from build123d import *

# Parameters (mm, degrees)
EXTRUDE_1_DEPTH        = 4
HOLE_WIZARD_M8_1_D     = 6.8
HOLE_WIZARD_M8_1_DEPTH = 19.75
HOLE_WIZARD_M8_1_TIP   = 2.042926105
FILLET_1_R             = 0.5


with BuildPart() as part:
    # 草图1 → 凸台-拉伸1 (new body)
    with BuildSketch(Plane.XY):
        Polygon((10.5, 14), (0, 0), (13.125, 0), (23.625, 14), align=None)
    extrude(amount=EXTRUDE_1_DEPTH)

    # M8 螺纹孔1
    with Locations(Plane(origin=(11.8125, 7, 4), x_dir=(1, 0, 0), z_dir=(0, 0, 1))):
        with Locations((0, 0)):
            Hole(HOLE_WIZARD_M8_1_D / 2, depth=HOLE_WIZARD_M8_1_DEPTH)
            with Locations((0, 0, -(HOLE_WIZARD_M8_1_DEPTH + HOLE_WIZARD_M8_1_TIP / 2))):  # 118° drill point
                Cone(0, HOLE_WIZARD_M8_1_D / 2, HOLE_WIZARD_M8_1_TIP, mode=Mode.SUBTRACT)

    # 圆角1
    fillet_1_edges = [part.edges().sort_by_distance(p)[0] for p in [
        (6.5625, 0, 4),
        (17.0625, 14, 4),
        (6.5625, 0, 0),
        (17.0625, 14, 0),
    ]]
    fillet(fillet_1_edges, radius=FILLET_1_R)


solid = part.part
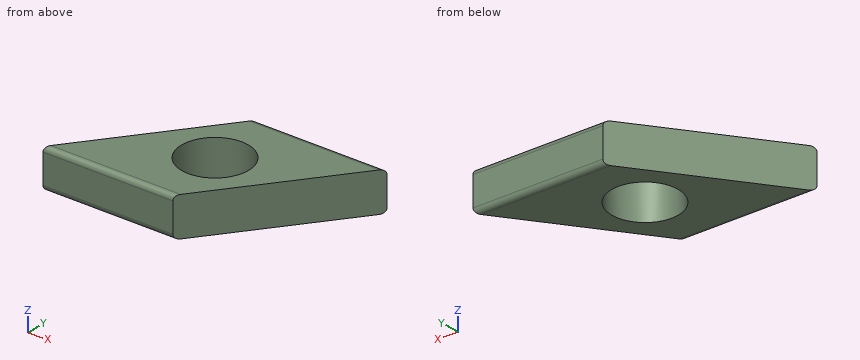
Here's how the part is built. I have some questions about the finished solid (model axes, mm). Coordinates: 2 decimals unless noted, no trailing zeros. Order: outer loops, then holes, each group sorted by start corner. A loop starts at its lowest first (then second) coordinate and runs counter-clockwise, first axis right, second up. Notation, with made-up numbers: M -13,27.5 L 4,27.5 A13 ccw 4,52.5 Z; hole C 27.5,54.5 d1. An arc over 180 degrees is marked long. Answer as CSV lines item,"result".
Item 1: If I drill on line 1 (X direction, y = 4, z = 2.1) (1 decimal); line 2 (Y direction, x = 10.25, z = 1.95); line 3 (Y direction, x = 6.5, z = 2.25), over which ranges is the centre line in solid material (lowest first)?
Results found:
line 1,"3 to 10.2, 13.4 to 16.1"
line 2,"0 to 3.98, 10.02 to 13.67"
line 3,"0 to 8.67"
Item 2: For pin 1 (1.5 mm diameter, centred on x = 5.5, z = 3, fed in from +Y), with a flat end and sliding along its axis, tell me the tip position at first contact or that it passes through.
Results found:
pin 1,"y = 8.33"
Item 3: Imagine slicing it at D-D on y = 8.75. Write out the boundary of the cut face in (x, z).
Results found:
outline,"M 6.56,0 L 8.9,0 L 8.9,4 L 6.56,4 Z; M 14.73,0 L 19.69,0 L 19.69,4 L 14.73,4 Z"
Item 4: Imagine slicing it at A-A on z = 3.05. Write out the boundary of the cut face in (x, y) (1 decimal), plus the area to 3 significant figures.
Results found:
outline,"M 0,0 L 13.1,0 L 23.6,14 L 10.5,14 Z; hole C 11.8,7 d6.8"
area,"147 mm2"
Item 5: Imagine slicing it at C-C on x = 6. Write out the boundary of the cut face in (y, z), plus the area to 3 significant figures.
Results found:
outline,"M 0,0.5 A0.5 ccw 0.5,0 L 8,0 L 8,4 L 0.5,4 A0.5 ccw 0,3.5 Z"
area,"31.9 mm2"
